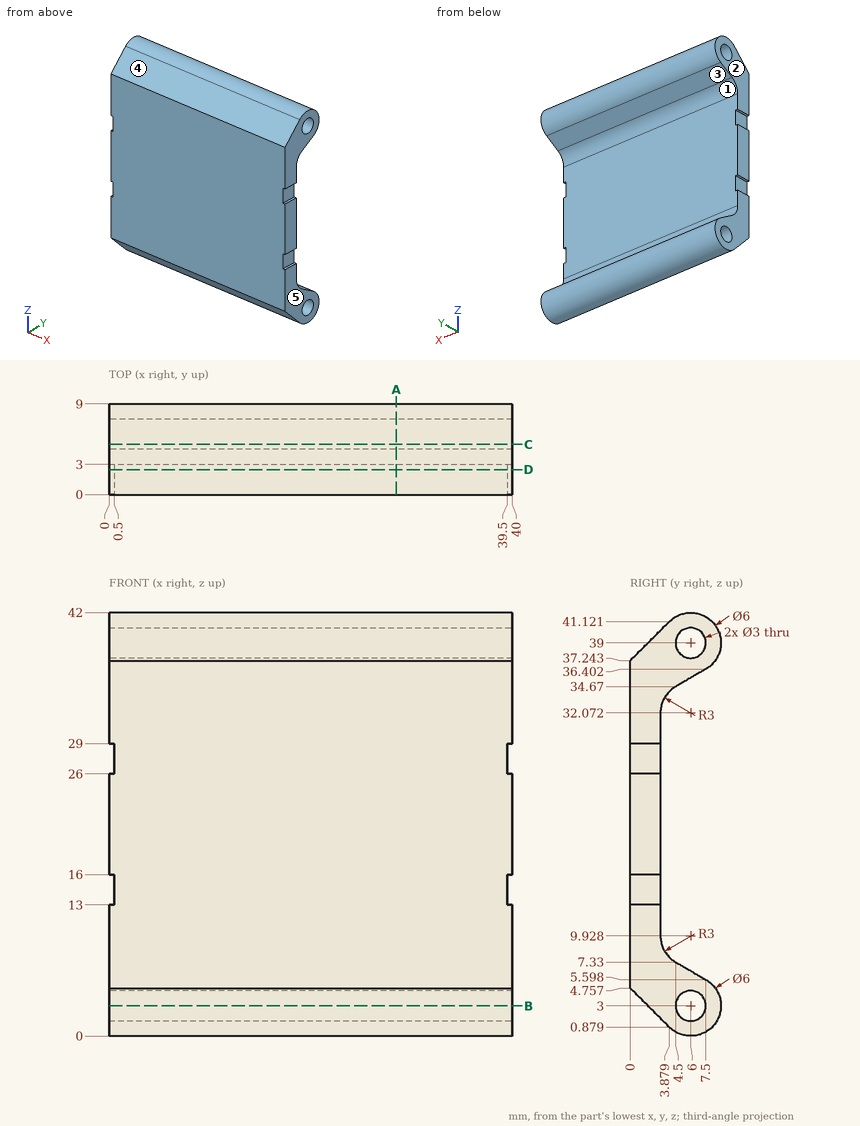
Geometry check sheet. Reference: drawing and pictorial views, mm from the part's lowest x, y, z. A direction names the side the tool comes from. Give positions to 0.01 mm unless a question says otherwise; leave off trailing zeros. Order: outer loops, then holes, each group sorted by start corner. A loop starts at its lowest first (then second) coordinate and runs counter-clockwise, first axis right, second up. Notation, with made-up numbers: (-11, 73.5) - (18, 73.5) arc R26 ccw to (18, 102.5) - close; hole circle Ø11 at (80.25, 6). An arc over 180 degrees is marked (long way). Answer as CSV lines item,"result". Start each with the question number.
Item 1: Section check A-A, the plane x = 28.5. Record the boundary of the cut face in (y, z).
Item 2: Section check B-B, the plane z = 3. Record the boundary of the cut face in (x, y).
Item 3: Access from +Z, -Z, +X, -X, +Y, -Y to the whole of each face (thin tool, end or side, straight path). Record for the marked faces 1 and 2.
Item 4: Material ranges on L1, parallel to Y at x = 4, z = 14; L2, parallel to Y at x = 18, z = 3; L3, parallel to Z at x = 34.5, y = 4 (1 decimal), recorded low to high.
Item 5: Mould release check, pull along Z, two halves, no side actions. Record for the marked faces 3, 4 and 5: released by +Z, released by -Z, zero draft, split by the parting line, or undercut.
Item 6: Section check C-C, the plane y = 5. Record the boundary of the cut face in (x, z).
Item 7: Gauge pin test, flat ends, axial feed: pin 1 (2.5 mm diameter, centred on y = 1, z = 27.5, fed in from -X); pin 2 (3 mm diameter, centred on y = 6, z = 27, fed in from +X); pin 3 (17.5 mm diameter, centred on x = 28.5, z = 19.5, fed in from +Y); pin 4 (1 mm diameter, centred on x = 28, y = 8, fed in from -Z). Record the tip position at first contact, or that the pin passes through.
Item 8: Section check D-D, the plane y = 2.5. Record the boundary of the cut face in (x, z).
Filled in:
1,outline,"(0, 4.76) - (3.88, 0.88) arc R3 ccw (long way) to (7.5, 5.6) - (4.5, 7.33) arc R3 cw to (3, 9.93) - (3, 32.07) arc R3 cw to (4.5, 34.67) - (7.5, 36.4) arc R3 ccw (long way) to (3.88, 41.12) - (0, 37.24) - close; hole circle Ø3 at (6, 3); hole circle Ø3 at (6, 39)"
2,outline,"(0, 1.76) - (40, 1.76) - (40, 4.5) - (0, 4.5) - close; (0, 7.5) - (40, 7.5) - (40, 9) - (0, 9) - close"
3,face 1,"+X, -X, +Y"
3,face 2,"+Z, -Z, -X, +Y, -Y"
4,L1,"0 to 3"
4,L2,"1.76 to 4.5, 7.5 to 9"
4,L3,"0.8 to 7.7, 34.3 to 41.2"
5,face 3,"undercut"
5,face 4,"released by +Z"
5,face 5,"zero draft"
6,outline,"(0, 0.17) - (40, 0.17) - (40, 1.88) - (0, 1.88) - close; (0, 4.12) - (40, 4.12) - (40, 7.04) - (0, 7.04) - close; (0, 34.96) - (40, 34.96) - (40, 37.88) - (0, 37.88) - close; (0, 40.12) - (40, 40.12) - (40, 41.83) - (0, 41.83) - close"
7,pin 1,"x = 0.5"
7,pin 2,"through"
7,pin 3,"y = 3"
7,pin 4,"z = 0.4"
8,outline,"(0, 2.26) - (40, 2.26) - (40, 13) - (39.5, 13) - (39.5, 16) - (40, 16) - (40, 26) - (39.5, 26) - (39.5, 29) - (40, 29) - (40, 39.74) - (0, 39.74) - (0, 29) - (0.5, 29) - (0.5, 26) - (0, 26) - (0, 16) - (0.5, 16) - (0.5, 13) - (0, 13) - close"
